```python
from build123d import *

# Parameters (mm, degrees)
SKETCH3_R           = 2
BOSS_EXTRUDE1_DEPTH = 2
BOSS_EXTRUDE2_DEPTH = 75
FILLET1_R           = 3


with BuildPart() as part:
    # Sketch3 → Boss-Extrude1 (new body)
    with BuildSketch(Plane.XY.offset(-3)):
        with BuildLine():
            Line((62.5, -66), (-47.5, -66))
            ThreePointArc((-47.5, -66), (-61.642135624, -60.142135624), (-67.5, -46))
            Line((-67.5, -46), (-67.5, -15))
            ThreePointArc((-67.5, -15), (-61.642135624, -0.857864376), (-47.5, 5))
            Line((-47.5, 5), (62.5, 5))
            ThreePointArc((62.5, 5), (76.642135624, -0.857864376), (82.5, -15))
            Line((82.5, -15), (82.5, -46))
            ThreePointArc((82.5, -46), (76.642135624, -60.142135624), (62.5, -66))
        make_face()
        with Locations((2.5, -12)):
            Circle(SKETCH3_R, mode=Mode.SUBTRACT)
        with Locations((12.5, -12)):
            Circle(SKETCH3_R, mode=Mode.SUBTRACT)
        with Locations((22.5, -12)):
            Circle(SKETCH3_R, mode=Mode.SUBTRACT)
        with Locations((32.5, -12)):
            Circle(SKETCH3_R, mode=Mode.SUBTRACT)
        with Locations((42.5, -12)):
            Circle(SKETCH3_R, mode=Mode.SUBTRACT)
        with Locations((-7.5, -12)):
            Circle(SKETCH3_R, mode=Mode.SUBTRACT)
        with Locations((-17.5, -12)):
            Circle(SKETCH3_R, mode=Mode.SUBTRACT)
        with Locations((-27.5, -12)):
            Circle(SKETCH3_R, mode=Mode.SUBTRACT)
        with Locations((7.5, -5)):
            Circle(SKETCH3_R, mode=Mode.SUBTRACT)
        with Locations((17.5, -5)):
            Circle(SKETCH3_R, mode=Mode.SUBTRACT)
        with Locations((27.5, -5)):
            Circle(SKETCH3_R, mode=Mode.SUBTRACT)
        with Locations((37.5, -5)):
            Circle(SKETCH3_R, mode=Mode.SUBTRACT)
        with Locations((47.5, -5)):
            Circle(SKETCH3_R, mode=Mode.SUBTRACT)
        with Locations((-2.5, -5)):
            Circle(SKETCH3_R, mode=Mode.SUBTRACT)
        with Locations((-12.5, -5)):
            Circle(SKETCH3_R, mode=Mode.SUBTRACT)
        with Locations((-22.5, -5)):
            Circle(SKETCH3_R, mode=Mode.SUBTRACT)
        with Locations((-32.5, -5)):
            Circle(SKETCH3_R, mode=Mode.SUBTRACT)
        with Locations((2.5, -26)):
            Circle(SKETCH3_R, mode=Mode.SUBTRACT)
        with Locations((12.5, -26)):
            Circle(SKETCH3_R, mode=Mode.SUBTRACT)
        with Locations((22.5, -26)):
            Circle(SKETCH3_R, mode=Mode.SUBTRACT)
        with Locations((32.5, -26)):
            Circle(SKETCH3_R, mode=Mode.SUBTRACT)
        with Locations((42.5, -26)):
            Circle(SKETCH3_R, mode=Mode.SUBTRACT)
        with Locations((-7.5, -26)):
            Circle(SKETCH3_R, mode=Mode.SUBTRACT)
        with Locations((-17.5, -26)):
            Circle(SKETCH3_R, mode=Mode.SUBTRACT)
        with Locations((-27.5, -26)):
            Circle(SKETCH3_R, mode=Mode.SUBTRACT)
        with Locations((7.5, -19)):
            Circle(SKETCH3_R, mode=Mode.SUBTRACT)
        with Locations((17.5, -19)):
            Circle(SKETCH3_R, mode=Mode.SUBTRACT)
        with Locations((27.5, -19)):
            Circle(SKETCH3_R, mode=Mode.SUBTRACT)
        with Locations((37.5, -19)):
            Circle(SKETCH3_R, mode=Mode.SUBTRACT)
        with Locations((47.5, -19)):
            Circle(SKETCH3_R, mode=Mode.SUBTRACT)
        with Locations((-2.5, -19)):
            Circle(SKETCH3_R, mode=Mode.SUBTRACT)
        with Locations((-12.5, -19)):
            Circle(SKETCH3_R, mode=Mode.SUBTRACT)
        with Locations((-22.5, -19)):
            Circle(SKETCH3_R, mode=Mode.SUBTRACT)
        with Locations((-32.5, -19)):
            Circle(SKETCH3_R, mode=Mode.SUBTRACT)
        with BuildLine():
            ThreePointArc((31.5, -53.323475383), (49, -48.2), (31.5, -43.076524617))
            ThreePointArc((31.5, -43.076524617), (23.5, -38.7), (15.5, -43.076524617))
            ThreePointArc((15.5, -43.076524617), (7.5, -38.7), (-0.5, -43.076524617))
            ThreePointArc((-0.5, -43.076524617), (-8.5, -38.7), (-16.5, -43.076524617))
            ThreePointArc((-16.5, -43.076524617), (-34, -48.2), (-16.5, -53.323475383))
            ThreePointArc((-16.5, -53.323475383), (-8.5, -57.7), (-0.5, -53.323475383))
            ThreePointArc((-0.5, -53.323475383), (7.5, -57.7), (15.5, -53.323475383))
            ThreePointArc((15.5, -53.323475383), (23.5, -57.7), (31.5, -53.323475383))
        make_face(mode=Mode.SUBTRACT)
    extrude(amount=-BOSS_EXTRUDE1_DEPTH)

    # Sketch5 → Boss-Extrude2 (add)
    with BuildSketch(Plane(origin=(0, 0, -5), x_dir=(-1, 0, 0), z_dir=(0, 0, -1))):
        with BuildLine():
            Line((67.5, -46), (67.5, -15))
            ThreePointArc((67.5, -15), (61.642135624, -0.857864376), (47.5, 5))
            Line((47.5, 5), (-62.5, 5))
            ThreePointArc((-62.5, 5), (-76.642135624, -0.857864376), (-82.5, -15))
            Line((-82.5, -15), (-82.5, -46))
            ThreePointArc((-82.5, -46), (-76.642135624, -60.142135624), (-62.5, -66))
            Line((-62.5, -66), (47.5, -66))
            ThreePointArc((47.5, -66), (61.642135624, -60.142135624), (67.5, -46))
        make_face()
        with BuildLine():
            Line((65.5, -46), (65.5, -15))
            ThreePointArc((65.5, -15), (60.227922061, -2.272077939), (47.5, 3))
            Line((47.5, 3), (-62.5, 3))
            ThreePointArc((-62.5, 3), (-75.227922061, -2.272077939), (-80.5, -15))
            Line((-80.5, -15), (-80.5, -46))
            ThreePointArc((-80.5, -46), (-75.227922061, -58.727922061), (-62.5, -64))
            Line((-62.5, -64), (47.5, -64))
            ThreePointArc((47.5, -64), (60.227922061, -58.727922061), (65.5, -46))
        make_face(mode=Mode.SUBTRACT)
    extrude(amount=BOSS_EXTRUDE2_DEPTH)

    # Fillet1
    fillet1_edges = [part.edges().sort_by_distance(p)[0] for p in [
        (82.5, -30.5, -3),
        (76.642135624, -60.142135624, -3),
        (7.5, -66, -3),
        (-61.642135624, -60.142135624, -3),
        (-60.227922061, -58.727922061, -5),
        (-65.5, -30.5, -5),
        (-60.227922061, -2.272077939, -5),
        (7.5, 3, -5),
        (75.227922061, -2.272077939, -5),
        (80.5, -30.5, -5),
        (75.227922061, -58.727922061, -5),
        (7.5, -64, -5),
        (-67.5, -30.5, -3),
        (-61.642135624, -0.857864376, -3),
        (7.5, 5, -3),
        (76.642135624, -0.857864376, -3),
    ]]
    fillet(fillet1_edges, radius=FILLET1_R)


solid = part.part
```
The listing builds one solid part. Answer for the finished solid, in the listing's coordinates (mm). A direction names the side the tool comes from. Coordinates: 2 decimals unless noted, no trailing zeros. Write each loop counter-clockwise with the first axis right and the second up, starting at its lowest first coordinate (ties: lowest second). Pieces come first, ordered by that corner, then holes. Notation, with made-up numbers: (47, 78) - (55, 78) arc R21 cw to (55, 83) - close; hole circle Ø3 at (68, -30.75). An arc over 180 degrees is marked (long way). Return JSON: item names as keys, results as strings. Group by question number.
Q1. For a pull along X with two mould halves and no side action, classify faces 1 (the flat face through (8, -66, -42)), 2 (the cylindrical face through (-18.974, -10.648, -3.986)), 3 (the flat face through (82.5, -30, -42)) as +X half, -X half, draft (parallel to the pull), parting line (faces both ways), or undercut.
Q2. The part is cut by section B-B on z = -38. Write down the section's boundary in (x, y).
Q3. The part is cut by section C-C on y = -19. State how many separate pieces and enclosed holes the cut face has, and give its area (3 significant figures).
Q4. Find the intervals of material crossed by line 1 along Y through (x, z) = (44, -29); line 2 along Y through (x, z) = (32.5, -4.05); line 3 along Y through (x, z) = (42.5, -3.7), in increasing order. Write a range as [from, to].
Q5. Flat-ended cylindrical pins translate along their axes: pin 1 Ø4.5 at (x, y) = (12.5, -26) entering from +Z; pin 2 Ø5 at (x, y) = (-32.5, -5) entering from -Z. Find the tip coordinate at first contact, or state that the pin passes through.
Q6. Which of the six approach directions +Z, -Z, +X, -X, +Y, -Y give full straight-line access (tool end or side, diameter ignored) to faces 4 (the cylindrical face through (75.087, -2.133, -43.496)), 5 (the cylindrical face through (-8.4, -38.7, -4)), 6 (the cylindrical face through (-61.797, -1.014, -42.482))?
Q7. The part is cut by section D-D on x = 56.5. Write down the section's boundary in (y, z), and give its area (3 significant figures).
Q8. The part is cut by section A-A on x = 2.5. Write down the section's boundary in (y, z), and give its area (3 significant figures).
Evaluation:
{
 "1": {"face 1": "draft", "face 2": "undercut", "face 3": "+X half"},
 "2": {"outline": "(-67.5, -46) arc R20 ccw to (-47.5, -66) - (62.5, -66) arc R20 ccw to (82.5, -46) - (82.5, -15) arc R20 ccw to (62.5, 5) - (-47.5, 5) arc R20 ccw to (-67.5, -15) - close; hole (-65.5, -46) arc R18 ccw to (-47.5, -64) - (62.5, -64) arc R18 ccw to (80.5, -46) - (80.5, -15) arc R18 ccw to (62.5, 3) - (-47.5, 3) arc R18 ccw to (-65.5, -15) - close"},
 "3": {"separate pieces": "10", "enclosed holes": "0", "area": "528 mm2"},
 "4": {"line 1": "y = [-66, -64], [3, 5]", "line 2": "y = [-65.28, -54.62], [-41.78, -28], [-24, -14], [-10, 4.28]", "line 3": "y = [-64.93, -57.21], [-39.19, -28], [-24, -14], [-10, 3.93]"},
 "5": {"pin 1": "stops at z = -3", "pin 2": "stops at z = -5"},
 "6": {"face 4": "-Z", "face 5": "+Z, -Z", "face 6": "+Z, -Z, -X, +Y"},
 "7": {"outline": "(-66, -80) - (-64, -80) - (-64, -8) arc R3 cw to (-61, -5) - (0, -5) arc R3 cw to (3, -8) - (3, -80) - (5, -80) - (5, -6) arc R3 ccw to (2, -3) - (-63, -3) arc R3 ccw to (-66, -6) - close", "area": "442 mm2"},
 "8": {"outline": "(-66, -80) - (-64, -80) - (-64, -8) arc R3 cw to (-61, -5) - (-56.28, -5) - (-56.28, -3) - (-63, -3) arc R3 ccw to (-66, -6) - close; (-40.12, -5) - (-28, -5) - (-28, -3) - (-40.12, -3) - close; (-24, -5) - (-14, -5) - (-14, -3) - (-24, -3) - close; (-10, -5) - (0, -5) arc R3 cw to (3, -8) - (3, -80) - (5, -80) - (5, -6) arc R3 ccw to (2, -3) - (-10, -3) - close", "area": "394 mm2"}
}
